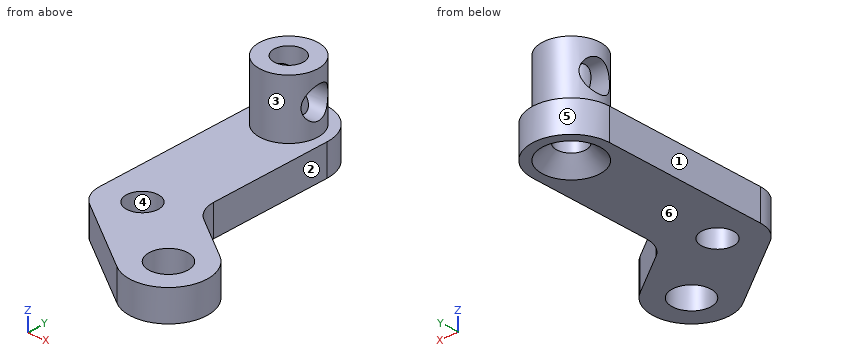
from build123d import *

# Parameters (mm, degrees)
SKETCH1_R                                       = 2
SKETCH1_R_2                                     = 1.65
BOSS_EXTRUDE1_DEPTH                             = 3.2
SKETCH5_R                                       = 3
BOSS_EXTRUDE2_DEPTH                             = 6
CSK_FOR_M3_FLAT_HEAD_MACHINE_SCREW2_D           = 3
CSK_FOR_M3_FLAT_HEAD_MACHINE_SCREW2_CSINK_D     = 6
CSK_FOR_M3_FLAT_HEAD_MACHINE_SCREW2_CSINK_ANGLE = 90
SKETCH8_R                                       = 1.6
CUT_EXTRUDE2_DEPTH                              = 16


with BuildPart() as part:
    # Sketch1 → Boss-Extrude1 (new body)
    with BuildSketch(Plane.XY):
        with BuildLine():
            Line((-4, -0.523005645), (-4, 16.35))
            ThreePointArc((-4, 16.35), (0, 20.35), (4, 16.35))
            Line((4, 16.35), (4, 3.661039513))
            ThreePointArc((4, 3.661039513), (4.341627544, 2.270695713), (5.288703922, 1.197005071))
            Line((5.288703922, 1.197005071), (9.931728104, -2.027620743))
            ThreePointArc((9.931728104, -2.027620743), (10.935379257, -7.594728104), (5.368271896, -8.598379257))
            Line((5.368271896, -8.598379257), (-2.711296078, -2.987040087))
            ThreePointArc((-2.711296078, -2.987040087), (-3.658372456, -1.913349445), (-4, -0.523005645))
        make_face()
        with Locations((7.65, -5.313)):
            Circle(SKETCH1_R, mode=Mode.SUBTRACT)
        Circle(SKETCH1_R_2, mode=Mode.SUBTRACT)
    extrude(amount=BOSS_EXTRUDE1_DEPTH)

    # Sketch5 → Boss-Extrude2 (add)
    with BuildSketch(Plane.XY.offset(3.2)):
        with Locations((0, 16.35)):
            Circle(SKETCH5_R)
    extrude(amount=BOSS_EXTRUDE2_DEPTH)

    # CSK for M3 Flat Head Machine Screw2 (through all)
    with Locations(Plane(origin=(0, 0, 0), x_dir=(-1, 0, 0), z_dir=(0, 0, -1))):
        with Locations((0, 16.35)):
            CounterSinkHole(CSK_FOR_M3_FLAT_HEAD_MACHINE_SCREW2_D / 2, CSK_FOR_M3_FLAT_HEAD_MACHINE_SCREW2_CSINK_D / 2, counter_sink_angle=CSK_FOR_M3_FLAT_HEAD_MACHINE_SCREW2_CSINK_ANGLE)

    # Sketch8 → Cut-Extrude2 (cut)
    with BuildSketch(Plane(origin=(4, 0, 0), x_dir=(0, 0, -1), z_dir=(1, 0, 0))):
        with Locations((-6.2, 16.5)):
            Circle(SKETCH8_R)
    extrude(amount=-CUT_EXTRUDE2_DEPTH, mode=Mode.SUBTRACT)


solid = part.part
The model under review builds one solid part; all positions refer to its coordinate system, in mm. Face numbers are marked on the shaded views. A direction names the side the tool comes from. Coordinates: 2 decimals unless noted, no trailing zeros. Write each loop counter-clockwise with the first axis right and the second up, starting at its lowest first coordinate (ties: lowest second). Pieces come first, ordered by that corner, then holes. Notation, with made-up numbers: M 14,-22 L 27,-22 A35 cw 27,17 Z; hole C 40,23 d6. An arc over 180 degrees is marked long. Put each result on its own line as item: value.
1) Wall thickness on probe 1 along Y at (x, z) = (0, 2.3); probe 2 along Y at (x, z) = (-1.25, 3); probe 3 along Z at (x, y) = (-0.5, -4): over which ranges is each line inside the solid? List them lowest first. Write a range as [from, to].
Computed:
probe 1: y = [-4.87, -1.65], [1.65, 14.85], [17.85, 20.35]
probe 2: y = [-4, -1.08], [1.08, 15.52], [17.18, 20.15]
probe 3: z = [0, 3.2]
2) Add section D-D on y = -5. Give the boundary of the cut face in (x, z).
Computed:
outline: M 0.19,0 L 5.67,0 L 5.67,3.2 L 0.19,3.2 Z; M 9.63,0 L 11.64,0 L 11.64,3.2 L 9.63,3.2 Z
3) Add section C-C on z = 2.75. Give the boundary of the cut face in (x, y).
Computed:
outline: M -4,-0.52 A3 ccw -2.71,-2.99 L 5.37,-8.6 A4 ccw 9.93,-2.03 L 5.29,1.2 A3 cw 4,3.66 L 4,16.35 A4 ccw -4,16.35 Z; hole C 0,0 d3.3; hole C 0,16.35 d3; hole C 7.65,-5.31 d4
4) Add section A-A on x = 7.65. Give the boundary of the cut face in (y, z).
Computed:
outline: M -9.31,0 L -7.31,0 L -7.31,3.2 L -9.31,3.2 Z; M -3.31,0 L -0.44,0 L -0.44,3.2 L -3.31,3.2 Z
5) Clearance check with flat-ended pins moving along their axes: pin 1 Ø5 at (x, y) = (7.65, -5.313) entering from +Z; pin 2 Ø2 at (y, z) = (14.5, 7) entering from -X; pin 3 Ø2.5 at (x, y) = (0, 16.35) entering from -Z; pin 4 Ø1 at (y, z) = (12.5, 1) entering from +X. State where each tip first meets the part, or that it passes through.
Computed:
pin 1: stops at z = 3.2
pin 2: stops at x = -2.85
pin 3: passes through
pin 4: stops at x = 4
6) Add section B-B on x = 0. Give the boundary of the cut face in (y, z).
Computed:
outline: M -4.87,0 L -1.65,0 L -1.65,3.2 L -4.87,3.2 Z; M 1.65,0 L 13.35,0 L 14.85,1.5 L 14.85,9.2 L 13.35,9.2 L 13.35,3.2 L 1.65,3.2 Z; M 17.85,1.5 L 19.35,0 L 20.35,0 L 20.35,3.2 L 19.35,3.2 L 19.35,9.2 L 17.85,9.2 L 17.85,7.06 A1.6 cw 17.85,5.34 Z
7) For the marked faces 1, 2 and 3, list the 3-axis set-ups (+Z, -Z, +X, -X, +Y, -Y) from which the entire face can be reached by the end or side of a thin tool; tool diameter is ignored.
Computed:
face 1: +Z, -Z, -X, +Y, -Y
face 2: +Z, -Z, +X, +Y
face 3: +Z
8) Draft analysis for pull direction X (two halves, no side actions). For the marked faces 4, 5 and 6, state which applies: released by +X, released by -X, zero draft, split by the parting line, or undercut.
Computed:
face 4: undercut
face 5: split by the parting line
face 6: zero draft
